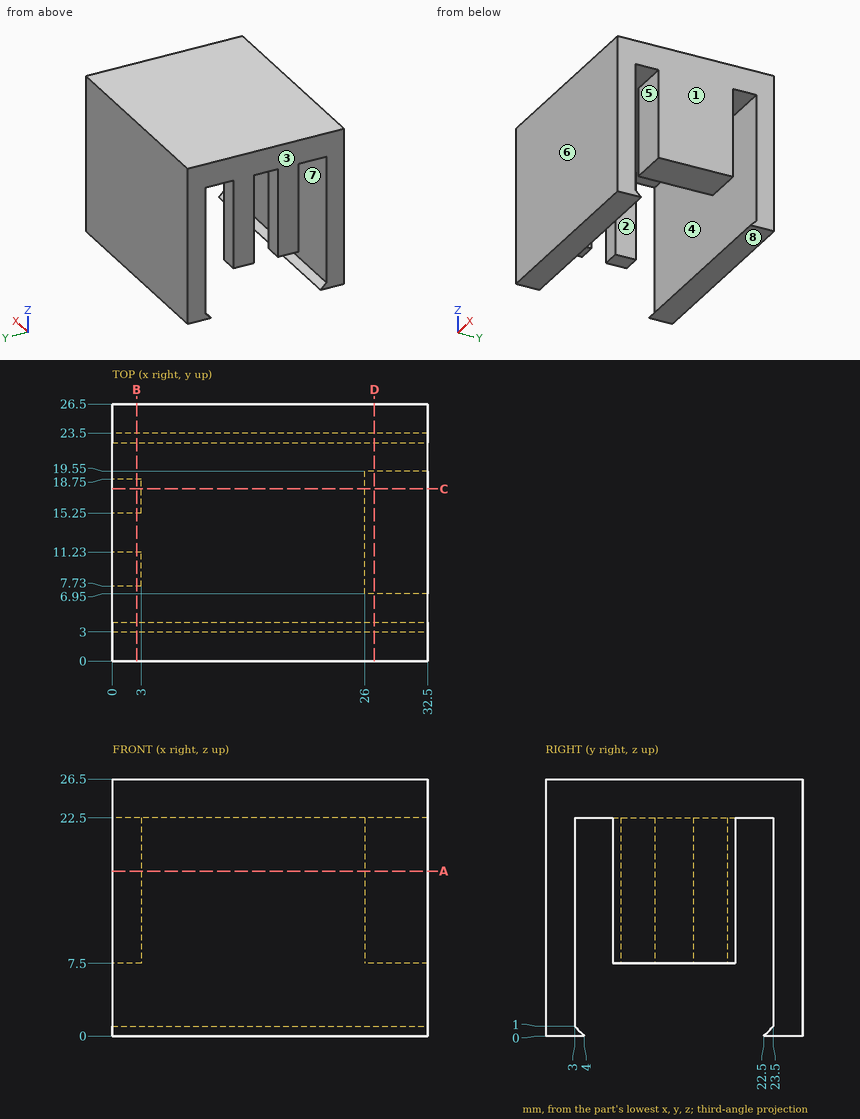
Could you check a few things on this drawing? It's one solid part, dimensions in mm from its lowest x, y, z. A direction names the side the tool comes from. Coordinates: 2 decimals unless noted, no trailing zeros. Write each loop counter-clockwise with the first axis right and the second up, starting at its lowest first coordinate (ties: lowest second). Pieces come first, ordered by that corner, then holes. Notation, with made-up numbers: (74.5, 31.5) - (130.5, 31.5) arc R19 cw to (130.5, 65.5) - close; hole circle Ø11 at (10.5, 60). An arc over 180 degrees is marked (long way). Put each result on its own line as item: value. Start each with the question number.
Q1. I want a section at C-C on y = 17.75. Write out the boundary of the cut face in (x, z), plus the area to 4 significant figures.
Q2. I want a section at A-A on z = 17. Write out the boundary of the cut face in (x, y).
Q3. I want a section at B-B on x = 2.5. Write out the boundary of the cut face in (y, z), plus the area to 3 significant figures.
Q4. Please list where these lines run through material, in increasing order: L1, parallel to Y at x = 31, z = 11.25; L2, parallel to Y at x = 4, z = 11.5; L3, parallel to X at y = 10.25, z = 19.5.
Q5. Which directions (+Z, -Z, +X, -X, +Y, -Y) give clear straight access to the entire face, cutting with the end or side of a thin tool? Please do the marked faces 1, 2, 3, 4 and 5.
Q6. Thinking about a two-plate mould opening in Z: for the marked faces 6, 7 and 8, which applies, pulls with the +Z half, pulls with the -Z half, needs draft (parallel to the pull), parting line crosses it, or undercut?
Q7. I want a section at D-D on x = 27. Write out the boundary of the cut face in (y, z), plus the area to 3 significant figures.
Q8. I'm going to push flat-ended pins straight in: P1, Ø1.5, axis at x = 1.5, y = 9, coming from the -Z side; P2, Ø5, axis at x = 5.5, y = 13, coming from the -Z side. Where does each tip first touch, or does it pass through?
Checks:
1. outline: (0, 7.5) - (3, 7.5) - (3, 22.5) - (26, 22.5) - (26, 7.5) - (32.5, 7.5) - (32.5, 26.5) - (0, 26.5) - close
1. area: 272.5 mm²
2. outline: (0, 0) - (32.5, 0) - (32.5, 3) - (0, 3) - close; (0, 7.73) - (3, 7.73) - (3, 11.23) - (0, 11.23) - close; (0, 15.25) - (3, 15.25) - (3, 18.75) - (0, 18.75) - close; (0, 23.5) - (32.5, 23.5) - (32.5, 26.5) - (0, 26.5) - close; (26, 6.95) - (32.5, 6.95) - (32.5, 19.55) - (26, 19.55) - close
3. outline: (0, 0) - (4, 0) - (3, 1) - (3, 22.5) - (7.73, 22.5) - (7.73, 7.5) - (11.23, 7.5) - (11.23, 22.5) - (15.25, 22.5) - (15.25, 7.5) - (18.75, 7.5) - (18.75, 22.5) - (23.5, 22.5) - (23.5, 1) - (22.5, 0) - (26.5, 0) - (26.5, 26.5) - (0, 26.5) - close
3. area: 347 mm²
4. L1: 0 to 3, 6.95 to 19.55, 23.5 to 26.5
4. L2: 0 to 3, 23.5 to 26.5
4. L3: 0 to 3, 26 to 32.5
5. face 1: +Z, -Z, +X, +Y, -Y
5. face 2: -Z
5. face 3: +Z, -Z, -X, +Y, -Y
5. face 4: +X, -X
5. face 5: -Z, +X, -X
6. face 6: needs draft
6. face 7: undercut
6. face 8: pulls with the -Z half
7. outline: (0, 0) - (4, 0) - (3, 1) - (3, 22.5) - (6.95, 22.5) - (6.95, 7.5) - (19.55, 7.5) - (19.55, 22.5) - (23.5, 22.5) - (23.5, 1) - (22.5, 0) - (26.5, 0) - (26.5, 26.5) - (0, 26.5) - close
7. area: 431 mm²
8. P1: z = 7.5
8. P2: z = 22.5
